```python
from build123d import *

# Parameters (mm, degrees)
SKETCH1_W           = 550
SKETCH1_H           = 350
BOSS_EXTRUDE1_DEPTH = 10
SKETCH2_R           = 12.5
BOSS_EXTRUDE2_DEPTH = 900
BOSS_EXTRUDE3_START = 910
SKETCH1_2_W         = 550
SKETCH1_2_H         = 350
BOSS_EXTRUDE3_DEPTH = 10
CUT_EXTRUDE1_START  = -920
SKETCH3_R           = 19.15
CUT_EXTRUDE1_DEPTH  = 10
LPATTERN1_COUNT     = 2
LPATTERN1_PITCH     = 120
MIRROR1_START       = 910
MIRROR1_OUTLINE_R   = 19.15
MIRROR1_DEPTH       = 10


# Read off the part's stored shape, not the designer's step: Mirror1
with BuildPart() as part:
    # Sketch1 → Boss-Extrude1 (new body)
    with BuildSketch(Plane(origin=(0, 0, 0), x_dir=(1, 0, 0), z_dir=(0, 1, 0))):
        Rectangle(SKETCH1_W, SKETCH1_H)
    extrude(amount=BOSS_EXTRUDE1_DEPTH)

    # Sketch2 → Boss-Extrude2 (add)
    with BuildSketch(Plane(origin=(0, 10, 0), x_dir=(1, 0, 0), z_dir=(0, 1, 0))):
        with Locations(Location((-230, 120, 0), (0, 0, 270))):
            Circle(SKETCH2_R)
        with Locations(Location((-230, -120, 0), (0, 0, 270))):
            Circle(SKETCH2_R)
        with Locations(Location((230, -120, 0), (0, 0, 270))):
            Circle(SKETCH2_R)
        with Locations(Location((230, 120, 0), (0, 0, 270))):
            Circle(SKETCH2_R)
    extrude(amount=BOSS_EXTRUDE2_DEPTH)

    # Sketch1<2> → Boss-Extrude3 (add)
    with BuildSketch(Plane(origin=(0, 0, 0), x_dir=(1, 0, 0), z_dir=(0, 1, 0)).offset(BOSS_EXTRUDE3_START)):
        Rectangle(SKETCH1_2_W, SKETCH1_2_H)
    extrude(amount=BOSS_EXTRUDE3_DEPTH)

    # Sketch3 → Cut-Extrude1 (cut)
    with BuildSketch(Plane(origin=(0, 920, 0), x_dir=(1, 0, 0), z_dir=(0, 1, 0)).offset(CUT_EXTRUDE1_START)):
        with Locations(Location((-120, 0, 0), (0, 0, 270))):
            Circle(SKETCH3_R)
    cut_extrude1 = extrude(amount=CUT_EXTRUDE1_DEPTH, mode=Mode.SUBTRACT)

    # LPattern1: Cut-Extrude1 ×2
    with Locations(*[(i * LPATTERN1_PITCH, 0, 0) for i in range(1, LPATTERN1_COUNT)]):
        add(cut_extrude1, mode=Mode.SUBTRACT)

    # Mirror1 outline → Mirror1 (cut)
    with BuildSketch(Plane(origin=(0, 0, 0), x_dir=(1, 0, 0), z_dir=(0, 1, 0)).offset(MIRROR1_START)):
        with Locations((-120, 0)):
            Circle(MIRROR1_OUTLINE_R)
    extrude(amount=MIRROR1_DEPTH, mode=Mode.SUBTRACT)


solid = part.part
```
CAD build for the part. Positions are in the model's coordinates, mm. A direction names the side the tool comes from. Coordinates: 2 decimals unless noted, no trailing zeros. Write each loop counter-clockwise with the first axis right and the second up, starting at its lowest first coordinate (ties: lowest second). Pieces come first, ordered by that corner, then holes.
(1) 3-axis set-ups, long thin cutter, end or side, ignore diameter. For faces 1 (the face through (-226.245, 453.7, 131.923)), 2 (the face through (-101.013, 4.93, -2.493)): which of +Z, -Z, +X, -X, +Y, -Y reach the whole face in a straight line?
(2) Flat gauge pin, fed straight in: pin 1 (1 mm diameter, centred on y = 572.5, z = -109, fed in from -X). Where does the tip first touch, or does it go through?
(3) Cut at A-A, the plane x = -120. List the corners of the cut face in (y, z).
(4) Drill centre lines: probe 1 along X at (y, z) = (5, 0); probe 2 along Y at (x, z) = (-87.5, -9.5); probe 3 along Z at (x, y) = (-120, 913.5). Where is each one in solid material? Low to high.
(5) Cut at B-B, the plane z = 69. List the corners of the cut face in (x, y).
(6) Cut at D-D, the plane z = 0. List the corners of the cut face in (x, y), and give its area (3 significant figures).
(7) Two-plate mould, pull along X, no slides. Class faces 3 (the face through (-4, 0, -41)), 4 (the face through (-11.65, 4.93, -15.2)): +X half, -X half, draft (parallel to the pull), parting line (faces both ways), or undercut.
(8) Cut at C-C, the plane x = 0. List the corners of the cut face in (y, z).
Geometry says:
1. face 1: none
1. face 2: +Y, -Y
2. pin 1: stops at x = -236.78
3. outline: (0, -175) - (10, -175) - (10, -19.15) - (0, -19.15) - close; (0, 19.15) - (10, 19.15) - (10, 175) - (0, 175) - close; (910, -175) - (920, -175) - (920, -19.15) - (910, -19.15) - close; (910, 19.15) - (920, 19.15) - (920, 175) - (910, 175) - close
4. probe 1: x = -275 to -139.15, -100.85 to -19.15, 19.15 to 275
4. probe 2: y = 0 to 10, 910 to 920
4. probe 3: z = -175 to -19.15, 19.15 to 175
5. outline: (-275, 0) - (275, 0) - (275, 10) - (-275, 10) - close; (-275, 910) - (275, 910) - (275, 920) - (-275, 920) - close
6. outline: (-275, 0) - (-139.15, 0) - (-139.15, 10) - (-275, 10) - close; (-275, 910) - (-139.15, 910) - (-139.15, 920) - (-275, 920) - close; (-100.85, 0) - (-19.15, 0) - (-19.15, 10) - (-100.85, 10) - close; (-100.85, 910) - (275, 910) - (275, 920) - (-100.85, 920) - close; (19.15, 0) - (275, 0) - (275, 10) - (19.15, 10) - close
6. area: 9,850 mm2
7. face 3: draft
7. face 4: undercut
8. outline: (0, -175) - (10, -175) - (10, -19.15) - (0, -19.15) - close; (0, 19.15) - (10, 19.15) - (10, 175) - (0, 175) - close; (910, -175) - (920, -175) - (920, 175) - (910, 175) - close
